from build123d import *

# Parameters (mm, degrees)
F0_R     = 30
F1_DEPTH = 1.5
F2_R     = 28.65
F3_DEPTH = 11.5
F4_R     = 30
F5_DEPTH = 1.5
F6_R     = 19
F7_DEPTH = 8
F8_R     = 4
F9_DEPTH = 22.501


with BuildPart() as f1:
    # F0 (on Front) → F1 (new body)
    with BuildSketch(Plane.XZ):
        Circle(F0_R)
    extrude(amount=F1_DEPTH)

    # F2 (on face) → F3 (join)
    with BuildSketch(Plane(origin=(0, 0, 0), x_dir=(-1, 0, 0), z_dir=(0, 1, 0))):
        Circle(F2_R)
    extrude(amount=F3_DEPTH)

    # F4 (on face) → F5 (join)
    with BuildSketch(Plane(origin=(0, 11.5, 0), x_dir=(-1, 0, 0), z_dir=(0, 1, 0))):
        Circle(F4_R)
    extrude(amount=F5_DEPTH)

    # F6 (on face) → F7 (join)
    with BuildSketch(Plane(origin=(0, 13, 0), x_dir=(-1, 0, 0), z_dir=(0, 1, 0))):
        Circle(F6_R)
    extrude(amount=F7_DEPTH)

    # F8 (on face) → F9 (cut, through all)
    with BuildSketch(Plane(origin=(0, 21, 0), x_dir=(-1, 0, 0), z_dir=(0, 1, 0))):
        Circle(F8_R)
    extrude(amount=-F9_DEPTH, mode=Mode.SUBTRACT)


solid = f1.part
Input: part model. Units: mm. Frame: model coordinates. A direction names the side the tool comes from. Give positions to 0.01 mm unless a question says otherwise; leave off trailing zeros. Write each loop counter-clockwise with the first axis right and the second up, starting at its lowest first coordinate (ties: lowest second). Pieces come first, ordered by that corner, then holes. Notation, with made-up numbers: M 67,41.5 L 125,41.5 A29 ccw 125,70.5 Z; hole C 24.5,72 d5. An arc over 180 degrees is marked long. Write item = value, one per line. Start each with the question number.
1) Draft query along X for faces 1 (the flat face through (0.3, 21, 4.5)), 2 (the cylindrical face through (0.867, 9.908, -3.905)), 3 (the cylindrical face through (-29.97, -0.74, 1.32)). Return one class per face: +X half, -X half, draft (parallel to the pull), parting line (faces both ways), or undercut.
2) Cut plane D-D on z = 17. Return the cut outline in (x, y), then the cut area to 3 significant figures.
3) First-contact query: pin 1 Ø6 at (y, z) = (16.5, -19) entering from -X; pin 2 Ø1.5 at (x, y) = (-1, 11.5) entering from +Z; pin 3 Ø1 at (x, z) = (-20.5, 15) entering from +Y; pin 4 Ø5 at (x, z) = (0, 0) entering from +Y. Flat tips, straight axial feed; report the tip coordinate or a pass-through.
4) Material intervals for line 1 along Z through (x, y) = (0, 10); line 2 along X through (y, z) = (7.5, 1.5); line 3 along X through (y, z) = (4.5, -1), sorted ascending. Write a range as [from, to].
5) Cut plane C-C on y = 17.5. Return the cut outline in (x, z).
6) Reachability of faces 4 (the flat face through (6, -1.5, 0)), 5 (the cylindrical face through (-8.767, 16.944, -16.856)), 6 (the flat face through (11, 0, -27)) from +Z, -Z, +X, -X, +Y, -Y: full face, straight path, thin tool, end or side. Return the list, or none.
7) Cut plane A-A on z = 0. Return the cut outline in (x, y), then the cut area to 3 significant figures.
8) Cut plane B-B on x = 0. Return the cut outline in (y, z).
Solved:
q1.face_1 = draft
q1.face_2 = undercut
q1.face_3 = parting line
q2.outline = M -24.72,-1.5 L 24.72,-1.5 L 24.72,0 L 23.06,0 L 23.06,11.5 L 24.72,11.5 L 24.72,13 L 8.49,13 L 8.49,21 L -8.49,21 L -8.49,13 L -24.72,13 L -24.72,11.5 L -23.06,11.5 L -23.06,0 L -24.72,0 Z
q2.area = 814 mm2
q3.pin_1 = -10.25
q3.pin_2 = 30
q3.pin_3 = 13
q3.pin_4 = through
q4.line_1 = [-28.65, -4], [4, 28.65]
q4.line_2 = [-28.61, -3.71], [3.71, 28.61]
q4.line_3 = [-28.63, -3.87], [3.87, 28.63]
q5.outline = C 0,0 d38; hole C 0,0 d8
q6.face_4 = +Z, -Z, +X, -X, -Y
q6.face_5 = +Y
q6.face_6 = none
q7.outline = M -30,-1.5 L -4,-1.5 L -4,21 L -19,21 L -19,13 L -30,13 L -30,11.5 L -28.65,11.5 L -28.65,0 L -30,0 Z; M 4,-1.5 L 30,-1.5 L 30,0 L 28.65,0 L 28.65,11.5 L 30,11.5 L 30,13 L 19,13 L 19,21 L 4,21 Z
q7.area = 963 mm2
q8.outline = M -1.5,-30 L 0,-30 L 0,-28.65 L 11.5,-28.65 L 11.5,-30 L 13,-30 L 13,-19 L 21,-19 L 21,-4 L -1.5,-4 Z; M -1.5,4 L 21,4 L 21,19 L 13,19 L 13,30 L 11.5,30 L 11.5,28.65 L 0,28.65 L 0,30 L -1.5,30 Z
